Verification items for the finished model (mm, model axes). Coordinates: 2 decimals unless noted, no trailing zeros. Order: outer loops, then holes, each group sorted by start corner. A loop starts at its lowest first (then second) coordinate and runs counter-clockwise, first axis right, second up. Notation, with made-up numbers: (77.25, 1) -> (117.25, 1) arc R24 cw to (117.25, 37) -> close; hole circle Ø9 at (40, 50). An arc over 180 degrees is marked (long way). Write each question's results on one line, items separated by ' | '. Start each with the question number.
(1) Cross-section at C-C on x = 30.5. Enter the section's corners in (y, z) (3 decimals), and give its area (3 significant figures).
(2) Draft check along X on faces 1 (the cylindrical face through (37.855, 1.565, -11.921)), 2 (the flat face through (-19, 0, -37)), 3 (the cylindrical face through (57.01, 1.57, 55.17)). Enter one of: +X half, -X half, draft (parallel to the pull), parting line (faces both ways), or undercut.
(3) Cross-section at B-B on z = -63. Enter the section's corners in (x, y) (3 decimals).
(4) Cross-section at D-D on z = -102. Enter the section's corners in (x, y) (3 decimals).
(5) Cross-section at A-A on y = 1.7. Enter the section's corners in (x, z) (1 decimal).
(6) Thickness scan on probe 1 along Z at (x, y) = (0, 2.45); probe 2 along X at (y, z) = (0.8, 16) (3 decimals); probe 3 along X at (y, z) = (2.1, -49.5) (3 decimals). Record the ranges inside material, lowest first. Write a range as [from, to].
```python
from build123d import *

# Parameters (mm, degrees)
SKETCH3_W           = 247.65
SKETCH3_H           = 247.65
BOSS_EXTRUDE5_DEPTH = 3.175
SKETCH1_R           = 39.6875
CUT_EXTRUDE3_DEPTH  = 4.175


with BuildPart() as part:
    # Sketch3 → Boss-Extrude5 (new body)
    with BuildSketch(Plane(origin=(0, 0, 0), x_dir=(1, 0, 0), z_dir=(0, 1, 0))):
        Rectangle(SKETCH3_W, SKETCH3_H)
    extrude(amount=BOSS_EXTRUDE5_DEPTH)

    # Sketch1 → Cut-Extrude3 (cut, through all)
    with BuildSketch(Plane(origin=(0, 0, 0), x_dir=(1, 0, 0), z_dir=(0, 1, 0))):
        with BuildLine():
            Line((-123.82627, -84.13877), (-123.82627, -123.82627))
            Line((-123.82627, -123.82627), (-84.13877, -123.82627))
            ThreePointArc((-84.13877, -123.82627), (-56.075469622, -56.075469622), (-123.82627, -84.13877))
        make_face()
        with Locations((0, -84.13877)):
            Circle(SKETCH1_R)
        with Locations((84.13877, 0)):
            Circle(SKETCH1_R)
        with Locations((0, 84.13877)):
            Circle(SKETCH1_R)
        with Locations((-84.13877, 0)):
            Circle(SKETCH1_R)
        with BuildLine():
            Line((123.82627, -123.82627), (123.82627, -84.13877))
            ThreePointArc((123.82627, -84.13877), (56.075469622, -56.075469622), (84.13877, -123.82627))
            Line((84.13877, -123.82627), (123.82627, -123.82627))
        make_face()
        with BuildLine():
            Line((-123.82627, 123.82627), (-123.82627, 84.13877))
            ThreePointArc((-123.82627, 84.13877), (-56.075469622, 56.075469622), (-84.13877, 123.82627))
            Line((-84.13877, 123.82627), (-123.82627, 123.82627))
        make_face()
        with BuildLine():
            Line((123.82627, 123.82627), (84.13877, 123.82627))
            ThreePointArc((84.13877, 123.82627), (56.075469622, 56.075469622), (123.82627, 84.13877))
            Line((123.82627, 84.13877), (123.82627, 123.82627))
        make_face()
        Circle(SKETCH1_R)
    extrude(amount=CUT_EXTRUDE3_DEPTH, mode=Mode.SUBTRACT)


solid = part.part
```
Results are:
1) outline: (0, -123.825) -> (3.175, -123.825) -> (3.175, -109.533) -> (0, -109.533) -> close; (0, -58.745) -> (3.175, -58.745) -> (3.175, -25.394) -> (0, -25.394) -> close; (0, 25.394) -> (3.175, 25.394) -> (3.175, 58.745) -> (0, 58.745) -> close; (0, 109.533) -> (3.175, 109.533) -> (3.175, 123.825) -> (0, 123.825) -> close | area: 303 mm2
2) face 1: undercut | face 2: draft | face 3: undercut
3) outline: (-123.825, 0) -> (-117.728, 0) -> (-117.728, 3.175) -> (-123.825, 3.175) -> close; (-50.549, 0) -> (-33.589, 0) -> (-33.589, 3.175) -> (-50.549, 3.175) -> close; (33.589, 0) -> (50.549, 0) -> (50.549, 3.175) -> (33.589, 3.175) -> close; (117.728, 0) -> (123.825, 0) -> (123.825, 3.175) -> (117.728, 3.175) -> close
4) outline: (-48.698, 0) -> (-35.441, 0) -> (-35.441, 3.175) -> (-48.698, 3.175) -> close; (35.441, 0) -> (48.698, 0) -> (48.698, 3.175) -> (35.441, 3.175) -> close
5) outline: (-123.8, -83.8) arc R39.7 cw (long way) to (-83.8, -123.8) -> (-0.3, -123.8) arc R39.7 cw (long way) to (0.3, -123.8) -> (83.8, -123.8) arc R39.7 cw (long way) to (123.8, -83.8) -> (123.8, -0.3) arc R39.7 cw (long way) to (123.8, 0.3) -> (123.8, 83.8) arc R39.7 cw (long way) to (83.8, 123.8) -> (0.3, 123.8) arc R39.7 cw (long way) to (-0.3, 123.8) -> (-83.8, 123.8) arc R39.7 cw (long way) to (-123.8, 83.8) -> (-123.8, 0.3) arc R39.7 cw (long way) to (-123.8, -0.3) -> close; hole circle Ø79.4 at (0, 0)
6) probe 1: z = [-44.45, -39.69], [39.69, 44.45] | probe 2: x = [-123.825, -120.458], [-47.819, -36.319], [36.319, 47.819], [120.458, 123.825] | probe 3: x = [-123.825, -103.51], [-64.767, -19.371], [19.371, 64.767], [103.51, 123.825]
